Geometry check sheet. Reference: drawing and pictorial views, mm from the part's lowest x, y, z. Coordinates: 2 decimals unless noted, no trailing zeros. Loops run counter-clockwise (first coordinate to the right, second up) from the corner with the lowest first, then second, coordinate; pieces in that order, holes last. Notation, with made-up numbers: (75, 65) - (107, 65) arc R16 ccw to (107, 75) - close; hole circle Ø2 at (38.25, 60.5). An arc over 180 degrees is marked (long way). Write each question's results on one line, items separated by ' | '. Start each with the question number.
1. Cross-section at C-C (y = 0.7). Record the cut outline in (x, z) (1 decimal).
2. Cross-section at B-B (z = 4.5). Record the cut outline in (x, y) (1 decimal).
3. Draft check along X on the marked faces 1, 2 and 3. Enter one of: released by +X, released by -X, zero draft, split by the parting line, or undercut.
4. Cross-section at A-A (x = 4.5). Record the cut outline in (y, z).
5. Cross-section at D-D (x = 7.25). Record the cut outline in (y, z).
6. Thickness scan on line 1 (Z direction, x = 2.5, y = 1.3); line 2 (X direction, y = 0.4, z = 3) (1 decimal); line 3 (Z direction, x = 5.5, y = 0.35) (1 decimal). Record the ranges inside material, lowest first. Write a range as [from, to].
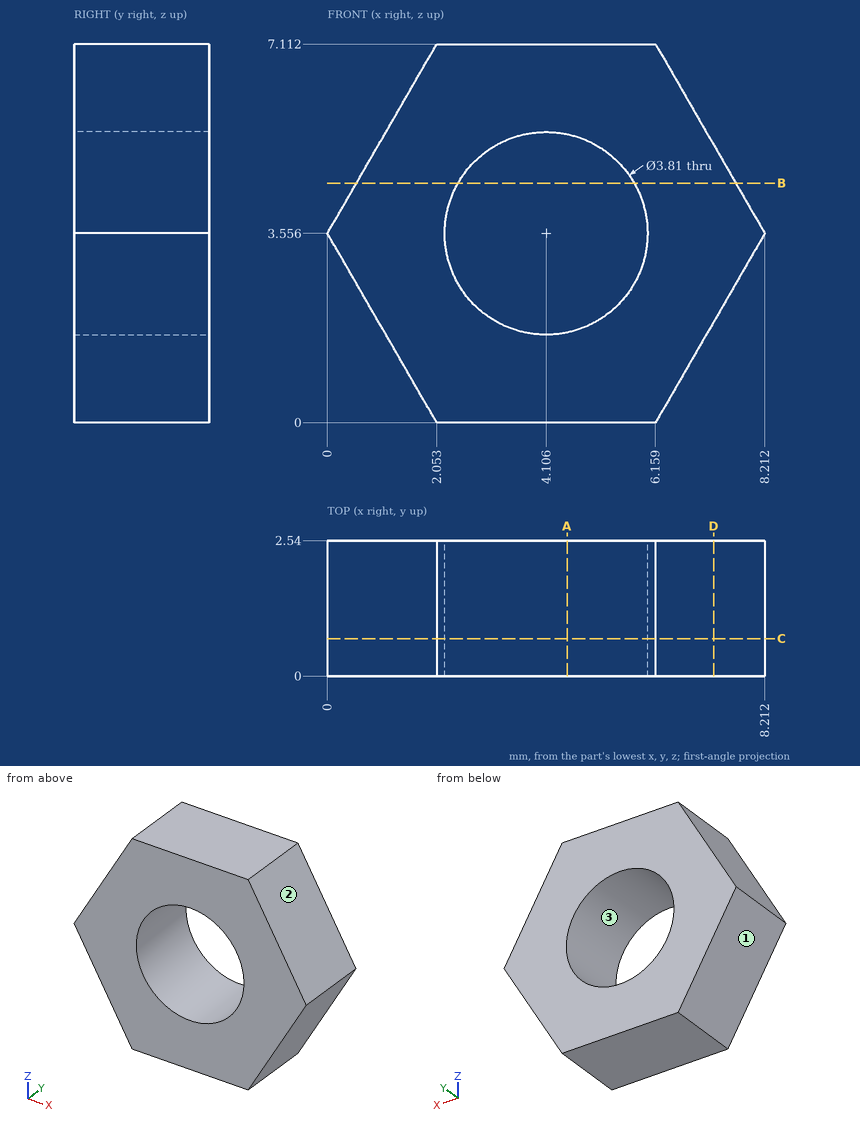
Established:
1) outline: (0, 3.6) - (2.1, 0) - (6.2, 0) - (8.2, 3.6) - (6.2, 7.1) - (2.1, 7.1) - close; hole circle Ø3.8 at (4.1, 3.6)
2) outline: (0.5, 0) - (2.5, 0) - (2.5, 2.5) - (0.5, 2.5) - close; (5.8, 0) - (7.7, 0) - (7.7, 2.5) - (5.8, 2.5) - close
3) face 1: released by -X | face 2: released by +X | face 3: undercut
4) outline: (0, 0) - (2.54, 0) - (2.54, 1.69) - (0, 1.69) - close; (0, 5.42) - (2.54, 5.42) - (2.54, 7.11) - (0, 7.11) - close
5) outline: (0, 1.89) - (2.54, 1.89) - (2.54, 5.22) - (0, 5.22) - close
6) line 1: [0, 2.53], [4.58, 7.11] | line 2: [0.3, 2.3], [5.9, 7.9] | line 3: [0, 2.3], [4.9, 7.1]
